```python
from build123d import *

# Parameters (mm, degrees)
SKETCH_1_W          = 20
SKETCH_1_H          = 40
EXTRUDE_1_DEPTH     = 10
FILLET_1_R          = 3
SKETCH_2_R          = 1.3
CUT_EXTRUDE_1_DEPTH = 15


with BuildPart() as part:
    # ｽｹｯﾁ1 → ﾎﾞｽ - 押し出し1 (new body)
    with BuildSketch(Plane.XY):
        Rectangle(SKETCH_1_W, SKETCH_1_H)
    extrude(amount=EXTRUDE_1_DEPTH)

    # ﾌｨﾚｯﾄ1
    fillet_1_edges = [part.edges().sort_by_distance(p)[0] for p in [
        (-10, 20, 5),
        (10, 20, 5),
        (10, -20, 5),
        (-10, -20, 5),
    ]]
    fillet(fillet_1_edges, radius=FILLET_1_R)

    # ｽｹｯﾁ2 → ｶｯﾄ - 押し出し1 (cut)
    with BuildSketch(Plane(origin=(10, 0, 0), x_dir=(0, 0, -1), z_dir=(1, 0, 0))):
        with Locations((-5, -15)):
            Circle(SKETCH_2_R)
        with Locations((-5, 5)):
            Circle(SKETCH_2_R)
    extrude(amount=-CUT_EXTRUDE_1_DEPTH, mode=Mode.SUBTRACT)


solid = part.part
```
CAD build for the part. Positions are in the model's coordinates, mm. A direction names the side the tool comes from. Give positions to 0.01 mm unless a question says otherwise; leave off trailing zeros. Order: outer loops, then holes, each group sorted by start corner. A loop starts at its lowest first (then second) coordinate and runs counter-clockwise, first axis right, second up.
(1) Flat gauge pin, fed straight in: pin 1 (1.3 mm diameter, centred on y = 4.5, z = 5, fed in from +X). Where does the tip first touch, or does it go through?
(2) Mould opens along Y. For faces 3 (the cylindrical face through (9.1, -19.14, 5.07)), 4 (the flat face through (-5, -15, 5)), 5 (the cylindrical face through (2.6, -15.5, 3.8)), 6 (the flat face through (0, 0, 10)) say: released by +Y, released by -Y, zero draft, split by the parting line, or undercut.
(3) Saw through at B-B, the plane y = -15. Give the cut face in (x, z).
(4) Saw through at C-C, the plane x = -2.5. Give the cut face in (y, z).
(5) Drill centre lines: L1, parallel to Y at x = 6.5, z = 5; L2, parallel to Y at x = -0.5, z = 4.25; L3, parallel to Y at x = 8.5, z = 0.5. Where is each one in solid material? Low to high.
(6) Tool access for faces 1 (the flat face through (0, 0, 0)), 2 (the cylindrical face through (2.605, 3.847, 4.4)): list every direction of +Z, -Z, +X, -X, +Y, -Y with a clear straight run to the whole face (end or side of a thin tool).
(7) Saw through at A-A, the plane z = 5. Give the cut face in (x, y).
Results found:
1. pin 1: stops at x = -5
2. face 3: released by -Y
2. face 4: undercut
2. face 5: undercut
2. face 6: zero draft
3. outline: (-10, 0) - (10, 0) - (10, 3.7) - (-5, 3.7) - (-5, 6.3) - (10, 6.3) - (10, 10) - (-10, 10) - close
4. outline: (-20, 0) - (20, 0) - (20, 10) - (-20, 10) - close; hole circle Ø2.6 at (-15, 5); hole circle Ø2.6 at (5, 5)
5. L1: y = -20 to -16.3, -13.7 to 3.7, 6.3 to 20
5. L2: y = -20 to -16.06, -13.94 to 3.94, 6.06 to 20
5. L3: y = -19.6 to 19.6
6. face 1: -Z, +X, -X, +Y, -Y
6. face 2: +X
7. outline: (-10, -17) arc R3 ccw to (-7, -20) - (7, -20) arc R3 ccw to (10, -17) - (10, -16.3) - (-5, -16.3) - (-5, -13.7) - (10, -13.7) - (10, 3.7) - (-5, 3.7) - (-5, 6.3) - (10, 6.3) - (10, 17) arc R3 ccw to (7, 20) - (-7, 20) arc R3 ccw to (-10, 17) - close
